Autodesk Inventor part; units mm, degrees
ref_plane "YZ Plane" through (0, 0, 0) normal (1, 0, 0) x (0, 1, 0)
ref_plane "XZ Plane" through (0, 0, 0) normal (0, 1, 0) x (-1, 0, 0)
ref_plane "XY Plane" through (0, 0, 0) normal (0, 0, 1) x (1, 0, 0)
sketch "Sketch1" plane through (0, 0, 0) normal (0, 0, 1) x (1, 0, 0)
  line L0 (0, 0) -> (34, 0)
  line L1 (34, 0) -> (34, 153)
  line L2 (34, 153) -> (0, 153)
  line L3 (0, 153) -> (0, 0)
  circle A0 centre (17, 7) radius 1.5
  circle A1 centre (17, 146) radius 1.5
  point P0 (17, 153)
  point P1 (17, 0)
  dimension "d0" = 34
  dimension "d1" = 153
  dimension "d2" = 3
  dimension "d4" = 7
  dimension "d5" = 3
  dimension "d6" = 7
extrude "Extrusion1" add sketch "Sketch1" along normal blind 5
sketch "Sketch2" plane through (0, 0, 0) normal (0, 0, -1) x (-1, 0, 0)
  line L0 (0, 153) -> (0, 0)
  line L1 (0, 138) -> (-34, 138)
  line L2 (-34, 138) -> (-34, 15)
  line L3 (-34, 15) -> (0, 15)
  line L4 (0, 15) -> (0, 138)
  line L5 (-34, 0) -> (-34, 153)
  point P0 (0, 76.5)
  dimension "d10" = 123
extrude "Extrusion2" add sketch "Sketch2" along normal blind 5
sketch "Sketch3" plane through (0, 0, 5) normal (0, 0, 1) x (1, 0, 0)
  line L0 (23, 33) -> (34, 33)
  line L1 (34, 33) -> (34, 120)
  line L2 (34, 120) -> (23, 120)
  line L3 (23, 120) -> (23, 33)
  line L4 (34, 0) -> (34, 153) construction
  line L5 (0, 15) -> (34, 15) construction
  line L6 (34, 138) -> (0, 138) construction
  line L7 (28.5, 33) -> (28.5, 15) construction
  line L8 (28.5, 120) -> (28.5, 138) construction
  dimension "d29" = 11
  dimension "d30" = 87
extrude "Extrusion3" cut sketch "Sketch3" against normal through all
sketch "Sketch4" plane through (0, 0, 5) normal (0, 0, 1) x (1, 0, 0)
  line L0 (17, 33) -> (6, 33)
  line L1 (6, 33) -> (6, 54)
  line L2 (6, 54) -> (17, 54)
  line L3 (17, 54) -> (17, 33)
  line L4 (23, 33) -> (23, 120)
  line L5 (0, 153) -> (0, 0)
  line L6 (6, 43.5) -> (0, 43.5)
  line L7 (17, 43.5) -> (23, 43.5)
  dimension "d17" = 11
  dimension "d18" = 21
extrude "Extrusion4" cut sketch "Sketch4" against normal through all
fillet "Fillet1" radius 2 4 edges at (6, 54, 0) (17, 54, 0) (17, 33, 0) (6, 33, 0)
sketch "Sketch6" plane through (0, 0, 5) normal (0, 0, 1) x (1, 0, 0)
  line L0 (21.5, 59) -> (1.5, 59)
  line L1 (1.5, 59) -> (1.5, 81)
  line L2 (1.5, 81) -> (21.5, 81)
  line L3 (21.5, 81) -> (21.5, 59)
  line L4 (17, 34) -> (17, 17) construction
  line L5 (8, 54) -> (15, 54) construction
  line L6 (1.5, 70) -> (0, 70) construction
  line L7 (0, 153) -> (0, 0) construction
  line L8 (21.5, 70) -> (23, 70) construction
  line L9 (23, 33) -> (23, 120)
  dimension "d23" = 20
  dimension "d24" = 22
  dimension "d25" = 5
extrude "Extrusion5" cut sketch "Sketch6" against normal through all
fillet "Fillet2" radius 2 4 edges at (21.5, 81, 0) (1.5, 81, 0) (1.5, 59, 0) (21.5, 59, 0)
sketch "Sketch7" plane through (0, 0, -5) normal (0, 0, -1) x (-1, 0, 0)
  line L0 (-21.5, 61) -> (-21.5, 79)
  arc A0 (-19.5, 81) -> (-21.5, 79) centre (-19.5, 79) ccw
  line L1 (-19.5, 81) -> (-3.5, 81)
  arc A1 (-1.5, 79) -> (-3.5, 81) centre (-3.5, 79) ccw
  line L2 (-1.5, 79) -> (-1.5, 61)
  arc A2 (-3.5, 59) -> (-1.5, 61) centre (-3.5, 61) ccw
  line L3 (-3.5, 59) -> (-19.5, 59)
  arc A3 (-21.5, 61) -> (-19.5, 59) centre (-19.5, 61) ccw
  line L4 (-17, 35) -> (-17, 52)
  arc A4 (-15, 54) -> (-17, 52) centre (-15, 52) ccw
  line L5 (-15, 54) -> (-8, 54)
  arc A5 (-6, 52) -> (-8, 54) centre (-8, 52) ccw
  line L6 (-6, 52) -> (-6, 35)
  arc A6 (-8, 33) -> (-6, 35) centre (-8, 35) ccw
  line L7 (-8, 33) -> (-15, 33)
  arc A7 (-17, 35) -> (-15, 33) centre (-15, 35) ccw
  line L8 (-23, 33) -> (-34, 33)
  line L9 (-34, 33) -> (-34, 15)
  line L10 (-34, 15) -> (0, 15)
  line L11 (0, 15) -> (0, 138)
  line L12 (0, 138) -> (-34, 138)
  line L13 (-34, 138) -> (-34, 120)
  line L14 (-34, 120) -> (-23, 120)
  line L15 (-23, 120) -> (-23, 33)
  point P0 (0, 0)
extrude "Extrusion6" add sketch "Sketch7" along normal blind 19
sketch "Sketch8" plane through (23, 33, 5) normal (0, 1, 0) x (1, 0, 0)
  line L0 (0, 0) -> (0, 29)
  line L1 (11, 0) -> (0, 0)
  line L2 (11, 29) -> (11, 0)
  line L3 (0, 29) -> (11, 29)
  line L4 (-23, 5) -> (11, 5)
  line L5 (0, 5) -> (11, 5)
extrude "Extrusion7" cut sketch "Sketch8" against normal through all contours L0 L3 L2 L4
sketch "Sketch9" plane through (23, 120, 5) normal (0, -1, 0) x (1, 0, 0)
  line L0 (11, -5) -> (-23, -5)
  line L1 (11, -5) -> (11, -29)
  line L2 (-23, -29) -> (11, -29)
  line L3 (-23, -5) -> (-23, -29)
  line L4 (0, 0) -> (0, -29)
  line L5 (0, 0) -> (0, -5)
  line L6 (0, -29) -> (0, -5)
  line L7 (-23, -29) -> (11, -29)
  line L8 (11, -29) -> (0, -29)
  line L9 (0, -29) -> (0, -5)
  line L10 (0, -5) -> (11, -5)
  line L11 (11, -5) -> (11, -29)
  point P0 (-23, -5)
extrude "Extrusion8" cut sketch "Sketch9" against normal through all contours L1 L2 L4 L0
properties part number "BP005" material "ABS Plastic"
Source: CAD feature listing. Evaluate the final solid. Frame: model axes, mm. A direction names the side the tool comes from. Round coordinates to 2 decimals unless told otherwise and drop trailing zeros. Loops run counter-clockwise (first coordinate to the right, second up) from the corner with the lowest first, then second, coordinate; pieces in that order, holes last.
Q1. Ray query, line 1 (X direction, y = 35, z = -6.25); line 2 (X direction, y = 146, z = 1); line 3 (X direction, y = 102, z = -16.75). Return the intervals inside material, ascending.
Q2. Section C-C, the plane z = -7.5. Return loops of the section in (x, y).
Q3. Mould query, pull axis X, two halves, no side actions, for faces 6 (the face through (17, 95, 5)), 7 (the face through (16.805, 144.513, 2.465)), 8 (the face through (17, 43, -9)), 9 (the face through (34, 17, 3)). Classes: pulls with the +X half, pulls with the -X half, needs draft (parallel to the pull), parting line crosses it, or undercut.
Q4. Section B-B, the plane x = 31. Return loops of the section in (y, z), plus the area to 3 significant figures.
Q5. Access query for faces 1 (the face through (29, 120, 3)), 2 (the face through (11, 138, -12)), 3 (the face through (12, 81, -9)), 4 (the face through (12, 91, -24)), 5 (the face through (12, 15, -12)). Directions: +Z, -Z, +X, -X, +Y, -Y. A direction counts if a zero-diameter tool reaches every point of the face in a straight line with its end or side. Return the directions, or none.
Q6. Section D-D, the plane x = 13. Return loops of the section in (y, z).
Q7. First-contact query: P1, Ø5, axis at x = 17, y = 7, coming from the -Z side; P2, Ø1.5, axis at y = 70.5, z = -16.5, coming from the +X side; P3, Ø7, axis at x = 6.5, z = -8, coming from the -Y side. Flat tips, straight axial feed; report the tip coordinate or a pass-through.
Q8. Section A-A, the plane y = 146. Return loops of the section in (x, z).
Solutions:
1. line 1: x = 0 to 6, 17 to 23
1. line 2: x = 0 to 15.5, 18.5 to 34
1. line 3: x = 0 to 23
2. outline: (0, 15) - (23, 15) - (23, 138) - (0, 138) - close; hole (1.5, 61) arc R2 ccw to (3.5, 59) - (19.5, 59) arc R2 ccw to (21.5, 61) - (21.5, 79) arc R2 ccw to (19.5, 81) - (3.5, 81) arc R2 ccw to (1.5, 79) - close; hole (6, 35) arc R2 ccw to (8, 33) - (15, 33) arc R2 ccw to (17, 35) - (17, 52) arc R2 ccw to (15, 54) - (8, 54) arc R2 ccw to (6, 52) - close
3. face 6: needs draft
3. face 7: undercut
3. face 8: undercut
3. face 9: pulls with the +X half
4. outline: (0, 0) - (33, 0) - (33, 5) - (0, 5) - close; (120, 0) - (153, 0) - (153, 5) - (120, 5) - close
4. area: 330 mm2
5. face 1: +Z, -Z, +X
5. face 2: -Z, +X, -X, +Y
5. face 3: +Z, -Z
5. face 4: -Z, +X, -X, +Y, -Y
5. face 5: -Z, +X, -X, -Y
6. outline: (0, 0) - (15, 0) - (15, -24) - (33, -24) - (33, 5) - (0, 5) - close; (54, -24) - (59, -24) - (59, 5) - (54, 5) - close; (81, -24) - (138, -24) - (138, 0) - (153, 0) - (153, 5) - (81, 5) - close
7. P1: stops at z = 0
7. P2: stops at x = 23
7. P3: stops at y = 15
8. outline: (0, 0) - (15.5, 0) - (15.5, 5) - (0, 5) - close; (18.5, 0) - (34, 0) - (34, 5) - (18.5, 5) - close
